Geometry check sheet. Reference: the model listing, model coordinates, mm. Give positions to 0.01 mm unless a question says otherwise; leave off trailing zeros. Loops run counter-clockwise (first coordinate to the right, second up) from the corner with the lowest first, then second, coordinate; pieces in that order, holes last. Notation, with made-up numbers: (66, 24) -> (97, 24) arc R10 ccw to (97, 40) -> close; hole circle Ø1 at (-28, 25). An arc over 180 degrees is marked (long way). One line per question, with ' | ' between items.
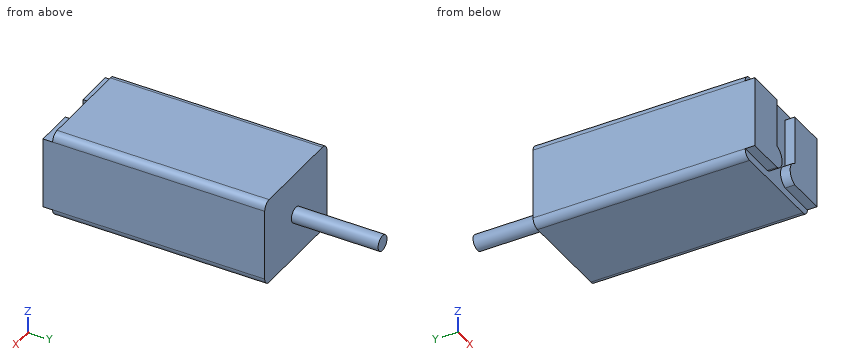
from build123d import *

# Parameters (mm, degrees)
SKETCH1_W           = 5.6
SKETCH1_H           = 4.5
BOSS_EXTRUDE1_DEPTH = 11
SKETCH2_R           = 0.4
BOSS_EXTRUDE2_DEPTH = 4.5
FILLET1_R           = 0.4
BOSS_EXTRUDE3_DEPTH = 0.5


with BuildPart() as part:
    # Sketch1 → Boss-Extrude1 (new body)
    with BuildSketch(Plane(origin=(0, 0, 0), x_dir=(1, 0, 0), z_dir=(0, 1, 0))):
        Rectangle(SKETCH1_W, SKETCH1_H)
    extrude(amount=BOSS_EXTRUDE1_DEPTH)

    # Sketch2 → Boss-Extrude2 (add)
    with BuildSketch(Plane(origin=(0, 11, 0), x_dir=(1, 0, 0), z_dir=(0, 1, 0))):
        with Locations(Location((0, 0, 0), (0, 0, 270))):
            Circle(SKETCH2_R)
    extrude(amount=BOSS_EXTRUDE2_DEPTH)

    # Fillet1
    fillet1_edges = [part.edges().sort_by_distance(p)[0] for p in [
        (2.8, 5.5, 2.25),
        (-2.8, 5.5, 2.25),
        (-2.8, 5.5, -2.25),
        (2.8, 5.5, -2.25),
    ]]
    fillet(fillet1_edges, radius=FILLET1_R)

    # Sketch3 → Boss-Extrude3 (add)
    with BuildSketch(Plane.XZ):
        with BuildLine():
            Line((-2.8, 1.85), (-0.8, 1.85))
            Line((-0.8, 1.85), (-0.8, -0.691387744))
            ThreePointArc((-0.8, -0.691387744), (-0.34347642, -1.270693872), (-0.8, -1.85))
            Line((-0.8, -1.85), (-2.8, -1.85))
            Line((-2.8, -1.85), (-2.8, 1.85))
        make_face()
        with BuildLine():
            Line((2.8, -1.85), (0.8, -1.85))
            ThreePointArc((0.8, -1.85), (0.384893305, -1.270693872), (0.8, -0.691387744))
            Line((0.8, -0.691387744), (0.8, 1.85))
            Line((0.8, 1.85), (2.8, 1.85))
            Line((2.8, 1.85), (2.8, -1.85))
        make_face()
    extrude(amount=BOSS_EXTRUDE3_DEPTH)


solid = part.part
Item 1: Scan lines: probe 1 along Y at (x, z) = (1.65, 0.7); probe 2 along X at (y, z) = (6.75, 1.9); probe 3 along Y at (x, z) = (-0.55, 0.2). Record each from-to range of solid material in increasing order.
Result:
probe 1: -0.5 to 11 | probe 2: -2.8 to 2.8 | probe 3: 0 to 11
Item 2: Sectioned sample at C-C (z = 1.15). Record the cut outline in (x, y).
Result:
outline: (-2.8, -0.5) -> (-0.8, -0.5) -> (-0.8, 0) -> (0.8, 0) -> (0.8, -0.5) -> (2.8, -0.5) -> (2.8, 11) -> (-2.8, 11) -> close
Item 3: Sectioned sample at A-A (z = 0). Record the cut outline in (x, y), plus the area to 3 significant figures.
Result:
outline: (-2.8, -0.5) -> (-0.8, -0.5) -> (-0.8, 0) -> (0.8, 0) -> (0.8, -0.5) -> (2.8, -0.5) -> (2.8, 11) -> (0.4, 11) -> (0.4, 15.5) -> (-0.4, 15.5) -> (-0.4, 11) -> (-2.8, 11) -> close | area: 67.2 mm2
Item 4: Sectioned sample at D-D (y = 12.5). Record the cut outline in (x, z).
Result:
outline: circle Ø0.8 at (0, 0)
Item 5: Depth check by flat-ended pin: pin 1 Ø2 at (x, y) = (1.5, 14) entering from +Z; pin 2 Ø0.6 at (x, y) = (1.5, -0.5) entering from +Z. Enter the tip coordinate at first touch or a pass-through.
Result:
pin 1: through | pin 2: z = 1.85
Item 6: Sectioned sample at B-B (x = 0). Record the cut outline in (y, z).
Result:
outline: (0, -2.25) -> (11, -2.25) -> (11, -0.4) -> (15.5, -0.4) -> (15.5, 0.4) -> (11, 0.4) -> (11, 2.25) -> (0, 2.25) -> close
